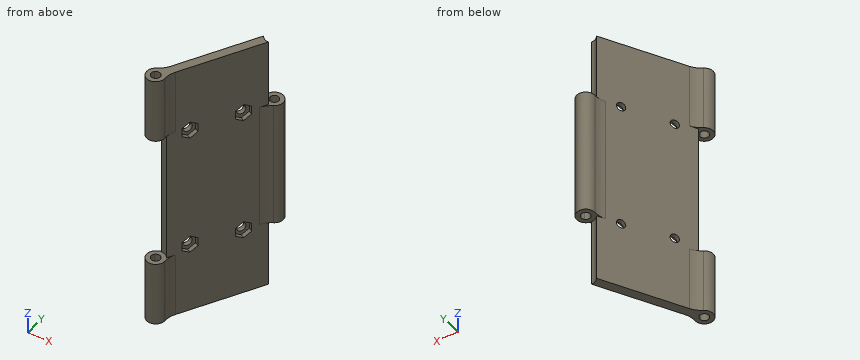
```python
from build123d import *

# Parameters (mm, degrees)
SKETCH2_R               = 1.5875
BOSS_EXTRUDE1_DEPTH     = 10
BOSS_EXTRUDE2_DEPTH     = 120
SKETCH4_R               = 4.0875
CUT_EXTRUDE1_DEPTH      = 30.5
CUT_EXTRUDE1_DEPTH_BACK = 30.5
SKETCH5_R               = 4.0875
CUT_EXTRUDE2_DEPTH      = 31
SKETCH6_R               = 4.0875
CUT_EXTRUDE3_DEPTH      = 31
FILLET1_R               = 10
SKETCH7_R               = 2
CUT_EXTRUDE4_DEPTH      = 4
CUT_EXTRUDE5_DEPTH      = 2


with BuildPart() as part:
    # Sketch2 → Boss-Extrude1 (new body)
    with BuildSketch(Plane.XY):
        with BuildLine():
            Line((0, -27.7495), (0, 0))
            Line((0, 0), (38.1, 0))
            ThreePointArc((38.1, 0), (-26.940768363, 26.940768363), (0, -38.1))
            Line((0, -38.1), (0, -30.9245))
            ThreePointArc((0, -30.9245), (-1.5875, -29.337), (0, -27.7495))
        make_face()
        with Locations((-25.406587271, 14.6685)):
            Circle(SKETCH2_R, mode=Mode.SUBTRACT)
        with Locations((25.406587271, 14.6685)):
            Circle(SKETCH2_R, mode=Mode.SUBTRACT)
        with BuildLine():
            Line((38.1, 0), (0, 0))
            Line((0, 0), (0, -27.7495))
            ThreePointArc((0, -27.7495), (1.122532015, -28.214467985), (1.5875, -29.337))
            ThreePointArc((1.5875, -29.337), (1.122532015, -30.459532015), (0, -30.9245))
            Line((0, -30.9245), (0, -38.1))
            ThreePointArc((0, -38.1), (26.940768363, -26.940768363), (38.1, 0))
        make_face()
    extrude(amount=BOSS_EXTRUDE1_DEPTH)


with BuildPart() as body_2:
    # Sketch3 → Boss-Extrude2 (new body)
    with BuildSketch(Plane.XY.offset(10)):
        with BuildLine():
            ThreePointArc((29.494087271, 14.6685), (24.324372064, 18.610132466), (21.892146477, 12.581309985))
            Line((21.892146477, 12.581309985), (23.37551462, 15.150578976))
            ThreePointArc((23.37551462, 15.150578976), (25.649272347, 16.741845172), (27.494087271, 14.6685))
            ThreePointArc((27.494087271, 14.6685), (27.323499399, 13.841998855), (26.839616236, 13.150578976))
            Line((26.839616236, 13.150578976), (25.356248092, 10.581309985))
            ThreePointArc((25.356248092, 10.581309985), (28.279033516, 11.760457906), (29.494087271, 14.6685))
        make_face()
        with BuildLine():
            Line((24.362837271, 12.86067197), (23.362837271, 11.128621162))
            ThreePointArc((23.362837271, 11.128621162), (24.324372064, 10.726867534), (25.356248092, 10.581309985))
            Line((25.356248092, 10.581309985), (26.839616236, 13.150578976))
            ThreePointArc((26.839616236, 13.150578976), (25.649272347, 12.595154828), (24.362837271, 12.86067197))
        make_face()
        with BuildLine():
            ThreePointArc((21.892146477, 12.581309985), (22.534141026, 11.760457906), (23.362837271, 11.128621162))
            Line((23.362837271, 11.128621162), (24.362837271, 12.86067197))
            ThreePointArc((24.362837271, 12.86067197), (23.489675143, 13.841998855), (23.37551462, 15.150578976))
            Line((23.37551462, 15.150578976), (21.892146477, 12.581309985))
        make_face()
        with BuildLine():
            Line((23.362837271, 11.128621162), (2.04375, -25.797121162))
            ThreePointArc((2.04375, -25.797121162), (2.872446245, -26.428957906), (3.514440794, -27.249809985))
            Line((3.514440794, -27.249809985), (25.356248092, 10.581309985))
            ThreePointArc((25.356248092, 10.581309985), (24.324372064, 10.726867534), (23.362837271, 11.128621162))
        make_face()
        with BuildLine():
            ThreePointArc((0.050339179, -25.249809985), (1.082215206, -25.395367534), (2.04375, -25.797121162))
            Line((2.04375, -25.797121162), (23.362837271, 11.128621162))
            ThreePointArc((23.362837271, 11.128621162), (22.534141026, 11.760457906), (21.892146477, 12.581309985))
            Line((21.892146477, 12.581309985), (0.050339179, -25.249809985))
        make_face()
        with BuildLine():
            ThreePointArc((-1.433028965, -27.819078976), (-0.242685076, -27.263654828), (1.04375, -27.52917197))
            Line((1.04375, -27.52917197), (2.04375, -25.797121162))
            ThreePointArc((2.04375, -25.797121162), (1.082215206, -25.395367534), (0.050339179, -25.249809985))
            Line((0.050339179, -25.249809985), (-1.433028965, -27.819078976))
        make_face()
        with BuildLine():
            Line((2.04375, -25.797121162), (1.04375, -27.52917197))
            ThreePointArc((1.04375, -27.52917197), (1.80782803, -28.29325), (2.0875, -29.337))
            ThreePointArc((2.0875, -29.337), (2.073345172, -29.579685076), (2.03107265, -29.819078976))
            Line((2.03107265, -29.819078976), (3.514440794, -27.249809985))
            ThreePointArc((3.514440794, -27.249809985), (2.872446245, -26.428957906), (2.04375, -25.797121162))
        make_face()
        with BuildLine():
            ThreePointArc((2.03107265, -29.819078976), (-1.04375, -31.14482803), (-1.433028965, -27.819078976))
            Line((-1.433028965, -27.819078976), (0.050339179, -25.249809985))
            ThreePointArc((0.050339179, -25.249809985), (-2.908042094, -32.209446245), (4.0875, -29.337))
            ThreePointArc((4.0875, -29.337), (3.941632466, -28.254784794), (3.514440794, -27.249809985))
            Line((3.514440794, -27.249809985), (2.03107265, -29.819078976))
        make_face()
    extrude(amount=BOSS_EXTRUDE2_DEPTH)

    # Sketch4 → Cut-Extrude1 (cut, two sides)
    with BuildSketch(Plane.XY.offset(70)) as cut_extrude1_sk:
        with Locations((0, -29.337)):
            Circle(SKETCH4_R)
    extrude(amount=CUT_EXTRUDE1_DEPTH, mode=Mode.SUBTRACT)
    extrude(cut_extrude1_sk.sketch, amount=-CUT_EXTRUDE1_DEPTH_BACK, mode=Mode.SUBTRACT)

    # Sketch5 → Cut-Extrude2 (cut)
    with BuildSketch(Plane(origin=(0, 0, 10), x_dir=(-1, 0, 0), z_dir=(0, 0, -1))):
        with Locations((-25.406587271, 14.6685)):
            Circle(SKETCH5_R)
    extrude(amount=-CUT_EXTRUDE2_DEPTH, mode=Mode.SUBTRACT)

    # Sketch6 → Cut-Extrude3 (cut)
    with BuildSketch(Plane.XY.offset(130)):
        with Locations((25.406587271, 14.6685)):
            Circle(SKETCH6_R)
    extrude(amount=-CUT_EXTRUDE3_DEPTH, mode=Mode.SUBTRACT)

    # Fillet1
    fillet1_edges = [body_2.edges().sort_by_distance(p)[0] for p in [
        (0.050339179, -25.249809985, 115.25),
        (3.514440794, -27.249809985, 115.25),
        (0.050339179, -25.249809985, 24.75),
        (3.514440794, -27.249809985, 24.75),
        (21.892146477, 12.581309985, 70),
        (25.356248092, 10.581309985, 70),
    ]]
    fillet(fillet1_edges, radius=FILLET1_R)

    # Sketch7 → Cut-Extrude4 (cut)
    with BuildSketch(Plane(origin=(10.971242828, -6.33425, 0), x_dir=(0, 0, 1), z_dir=(-0.866025404, 0.5, 0))):
        with Locations((40.981352926, 11.266107412)):
            Circle(SKETCH7_R)
        with Locations((42.485061868, -11.733892588)):
            Circle(SKETCH7_R)
        with Locations((98.981352926, -11.733892588)):
            Circle(SKETCH7_R)
        with Locations((98.981352926, 11.266107412)):
            Circle(SKETCH7_R)
    extrude(amount=-CUT_EXTRUDE4_DEPTH, mode=Mode.SUBTRACT)

    # Sketch8 → Cut-Extrude5 (cut)
    with BuildSketch(Plane(origin=(14.435344443, -8.33425, 0), x_dir=(0, 0, -1), z_dir=(0.866025404, -0.5, 0))):
        Polygon((-37.02188478, 11.266107412), (-39.001618853, 14.695107412), (-42.961086999, 14.695107412), (-44.940821072, 11.266107412), (-42.961086999, 7.837107412), (-39.001618853, 7.837107412), align=None)
        Polygon((-38.525593722, -11.733892588), (-40.505327795, -8.304892588), (-44.464795941, -8.304892588), (-46.444530014, -11.733892588), (-44.464795941, -15.162892588), (-40.505327795, -15.162892588), align=None)
        Polygon((-95.02188478, 11.266107412), (-97.001618853, 14.695107412), (-100.961086999, 14.695107412), (-102.940821072, 11.266107412), (-100.961086999, 7.837107412), (-97.001618853, 7.837107412), align=None)
        Polygon((-95.02188478, -11.733892588), (-97.001618853, -8.304892588), (-100.961086999, -8.304892588), (-102.940821072, -11.733892588), (-100.961086999, -15.162892588), (-97.001618853, -15.162892588), align=None)
    extrude(amount=-CUT_EXTRUDE5_DEPTH, mode=Mode.SUBTRACT)


solid = body_2.part
```
Design review of the part built by this model. Coordinates are the model's own, in mm. Coordinates: 2 decimals unless noted, no trailing zeros. Write each loop counter-clockwise with the first axis right and the second up, starting at its lowest first coordinate (ties: lowest second). Pieces come first, ordered by that corner, then holes.
1) To check wall thickness, follow L1, parallel to Y at x = 0, z = 118.5; L2, parallel to X at y = -30, z = 16; L3, parallel to Z at x = 16, y = 2. State the ranges of each line that lie inside material, in increasing order.
2) Add section A-A (z = 58). Write out the cut boundary in (x, y) (1 decimal), plus the area to 3 significant figures.
3) Insertion check: pin 1 (1 mm diameter, centred on y = -7.5, z = 83.5, fed in from +X); pin 2 (2 mm diameter, centred on x = 16.5, z = 96.5, fed in from +Y); pin 3 (7.5 mm diameter, centred on x = 26.5, y = 16, fed in from -Z). Each pin has a flat end and moves straight along its axis. Give the tip position at first contact, or say it passes through.
4) Add section B-B (y = -3). Write out the cut boundary in (x, z).
Check result:
1. L1: y = -33.42 to -31.42, -27.25 to -24.37
1. L2: x = -4.03 to -1.98, 1.98 to 4.03
1. L3: z = 10 to 39.7, 42.26 to 97.7, 100.26 to 130
2. outline: (0.1, -25.2) arc R4.1 cw to (3.5, -27.2) - (23.4, 7.3) arc R10 cw to (27.4, 11.1) arc R4.1 ccw (long way) to (21.3, 14.6) arc R10 cw to (20, 9.3) - close; hole circle Ø4.2 at (25.4, 14.7)
2. area: 213 mm2
3. pin 1: stops at x = 15.21
3. pin 2: stops at y = 4.97
3. pin 3: stops at z = 41
4. outline: (12.9, 10) - (17.52, 10) - (17.52, 130) - (12.9, 130) - close
